Design review of the part built by this model. Coordinates are the model's own, in mm. Round coordinates to 2 decimals unless told otherwise and drop trailing zeros. Write each loop counter-clockwise with the first axis right and the second up, starting at its lowest first coordinate (ties: lowest second). Pieces come first, ordered by that corner, then holes. Notation, with made-up numbers: (40.5, 22) -> (57.5, 22) arc R15 ccw to (57.5, 40) -> close; hole circle Ø3 at (-8, -22.5). An arc over 180 degrees is marked (long way). Write item = value, one per line. Start each with the question number.
Item 1: To check wall thickness, follow L1, parallel to Y at x = -32.5, z = 10.75; L2, parallel to X at y = -150, z = 5.5; L3, parallel to X at y = -63, z = 10.75. State the ranges of each line that lie inside material, in increasing order.
Item 2: Add section B-B, the plane z = 6. State how many separate pieces and enclosed holes the cut face has, then the cut area to 3 significant figures.
Item 3: Add section D-D, the plane x = -87.5. State the section outline as (y, z) points, then the cut area to 3 significant figures.
Item 4: Add section C-C, the plane y = -33.5. State the section outline as (x, z) points.
Item 5: Add section A-A, the plane x = -13. State the section outline as (y, z) points, then the cut area to 3 significant figures.
from build123d import *

# Parameters (mm, degrees)
F0_W     = 645
F0_H     = 430
F1_DEPTH = 15
F3_D     = 10.3
F4_R     = 8.5
F5_DEPTH = 15


with BuildPart() as f1:
    # F0 (on Top) → F1 (new body)
    with BuildSketch(Plane.XY):
        Rectangle(F0_W, F0_H)
        Polygon((-132.5, 120), (-117.5, 135), (207.5, 135), (222.5, 120), (222.5, -120), (207.5, -135), (-117.5, -135), (-132.5, -120), align=None, mode=Mode.SUBTRACT)
    extrude(amount=F1_DEPTH)

    # F3 (through all)
    with Locations(Plane(origin=(0, 0, 0), x_dir=(1, 0, 0), z_dir=(0, 0, -1))):
        with Locations((-297.5, -150), (-297.5, 150), (-157.5, -150), (-157.5, 0), (-157.5, 150), (-32.5, 185), (57.5, 185), (212.5, 185), (302.5, 185), (302.5, -185), (212.5, -185), (57.5, -185), (-32.5, -185), (-269.5, 0)):
            Hole(F3_D / 2)

    # F4 (on Top) → F5 (cut, through all)
    with BuildSketch(Plane.XY):
        with Locations((-87.5, 185)):
            Circle(F4_R)
        with Locations((162.5, 185)):
            Circle(F4_R)
        with Locations((162.5, -185)):
            Circle(F4_R)
        with Locations((-87.5, -185)):
            Circle(F4_R)
    extrude(amount=F5_DEPTH, mode=Mode.SUBTRACT)


solid = f1.part
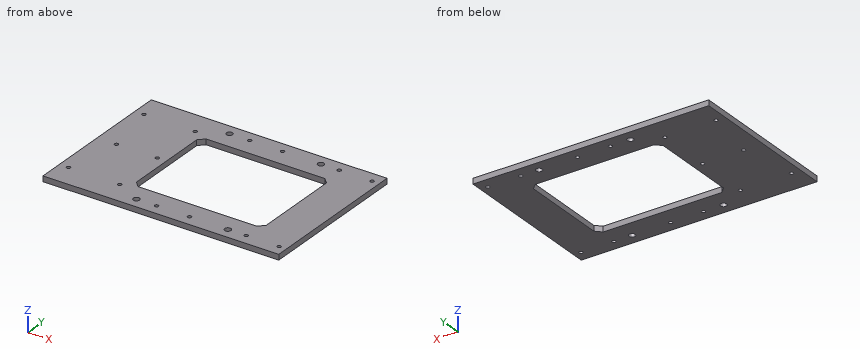
Result set:
q1.L1 = -215 to -190.15, -179.85 to -135, 135 to 179.85, 190.15 to 215
q1.L2 = -322.5 to -302.65, -292.35 to -162.65, -152.35 to 322.5
q1.L3 = -322.5 to -132.5, 222.5 to 322.5
q2.separate_pieces = 1
q2.enclosed_holes = 19
q2.area = 180,000 mm²
q3.outline = (-215, 0) -> (-193.5, 0) -> (-193.5, 15) -> (-215, 15) -> close; (-176.5, 0) -> (-135, 0) -> (-135, 15) -> (-176.5, 15) -> close; (135, 0) -> (176.5, 0) -> (176.5, 15) -> (135, 15) -> close; (193.5, 0) -> (215, 0) -> (215, 15) -> (193.5, 15) -> close
q3.area = 1,890 mm²
q4.outline = (-322.5, 0) -> (-132.5, 0) -> (-132.5, 15) -> (-322.5, 15) -> close; (222.5, 0) -> (322.5, 0) -> (322.5, 15) -> (222.5, 15) -> close
q5.outline = (-215, 0) -> (-135, 0) -> (-135, 15) -> (-215, 15) -> close; (135, 0) -> (215, 0) -> (215, 15) -> (135, 15) -> close
q5.area = 2,400 mm²
